Input: part model. Units: mm. Frame: model coordinates. A direction names the side the tool comes from. Coordinates: 2 decimals unless noted, no trailing zeros. Order: outer loops, then holes, each group sorted by start corner. A loop starts at its lowest first (then second) coordinate and runs counter-clockwise, first axis right, second up. Notation, with made-up numbers: (42.5, 46.25) -> (93.5, 46.25) arc R21 cw to (93.5, 65.25) -> close; hole circle Ø9 at (26.5, 82). An arc over 180 degrees is marked (long way). Use CSV: the item, a comma, the result in double quotes. Start each with the question number.
```python
from build123d import *

# Parameters (mm, degrees)
F2_SIZE = 0.5
F3_SIZE = 1.5
F4_SIZE = 1.82


with BuildPart() as f1:
    # F0 (on Front) → F1 (revolve)
    with BuildSketch(Plane.XZ):
        Polygon((0, 8), (0, 0), (77, 0), (77, 8), (46.45, 8), (46.45, 23), (41.45, 23), (41.45, 45.9), (29.5, 45.9), (29.5, 23.5), (10, 23.5), (10, 8), align=None)
    revolve(axis=Axis((38.5, 0, 0), (-1, 0, 0)))

    # F2
    f2_edges = [f1.edges().sort_by_distance(p)[0] for p in [
        (0, 0, -8),
        (10, 0, -23.5),
        (46.45, 0, -23),
    ]]
    chamfer(f2_edges, length=F2_SIZE)

    # F3
    f3_edges = [f1.edges().sort_by_distance(p)[0] for p in [
        (77, 0, -8),
    ]]
    chamfer(f3_edges, length=F3_SIZE)

    # F4
    f4_edges = [f1.edges().sort_by_distance(p)[0] for p in [
        (41.45, 0, -45.9),
        (29.5, 0, -45.9),
    ]]
    chamfer(f4_edges, length=F4_SIZE)


solid = f1.part
```
1. Access query for faces 1 (the face through (41.45, -19, -19)), 2 (the face through (77, 0, 0)), 3 (the face through (10, 0, 10)). Directions: +Z, -Z, +X, -X, +Y, -Y. A direction counts if a zero-diameter tool reaches every point of the face in a straight line with its end or side. Return the directions, or none.
2. Section D-D on x = 36. Return loops of the section in (y, z).
3. Contact query for flat-ended pins moving along their axis: P1, Ø23, axis at y = 9.5, z = 10, coming from the -X side; P2, Ø4, axis at x = 30.5, z = 7, coming from the +Y side; P3, Ø10, axis at x = 41, z = 4.5, coming from the -Y side; P4, Ø1, axis at x = 44, z = 13.5, coming from the +Y side. Output: stop coordinate, or through.
4. Section C-C on x = 55.5. Return loops of the section in (y, z), then the cut area to 3 significant figures.
5. Material intervals for line 1 along X through (y, z) = (-2, -41); line 2 along X through (y, z) = (-14, 2); line 3 along Y through (x, z) = (44, 1), sorted ascending.
Values follow:
1,face 1,"+X"
1,face 2,"+Z, -Z, +X, +Y, -Y"
1,face 3,"-X"
2,outline,"circle Ø91.8 at (0, 0)"
3,P1,"stops at x = 0"
3,P2,"stops at y = 45.61"
3,P3,"stops at y = -45.9"
3,P4,"stops at y = 18.97"
4,outline,"circle Ø16 at (0, 0)"
4,area,"201 mm2"
5,line 1,"x = 29.5 to 41.45"
5,line 2,"x = 10 to 46.45"
5,line 3,"y = -22.98 to 22.98"
